from build123d import *

# Parameters (mm, degrees)
F4_START = 28
F4_DEPTH = 22
F6_START = -28
F5_W     = 60
F5_H     = 60
F6_DEPTH = 72


with BuildPart() as f2:
    # F1 (on Front) → F2 (revolve)
    with BuildSketch(Plane.XZ):
        with BuildLine():
            Line((-30, 0), (30, 0))
            ThreePointArc((30, 0), (0, 30), (-30, 0))
        make_face()
    revolve(axis=Axis((0, 0, 0), (1, 0, 0)))

    # F3 (on Top) → F4 (cut)
    with BuildSketch(Plane.XY.offset(F4_START)):
        Polygon((-9.1697992757, 6.1277179047), (-9.1697992757, -4.0975827724), (-6.1292964965, -5.6231399067), (-6.1292964965, 4.3796850368), (0, 7.6826182194), (5.4949265905, 4.3796850368), (5.4949265905, -2.3808549158), (-0.4257261462, -5.8186533861), (-4.6656387858, -3.3751989249), (-4.6656387858, -6.7009669729), (0, -9.1569181532), (8.5351010785, -4.193849396), (8.5351010785, 6.2439450994), (-0.4188895691, 11.2581793219), align=None)
        Polygon((-4.7212797217, 3.3881671261), (-4.7212797217, -1.4694901183), (0, -4.0975827724), (4.0084240027, -1.328688697), (4.0084240027, 3.3881671261), (0, 6.1423662119), align=None)
    extrude(amount=F4_DEPTH, mode=Mode.SUBTRACT)

    # F5 (on Top) → F6 (cut)
    with BuildSketch(Plane.XY.offset(F6_START)):
        with Locations((1.9770637155, -0.5929265171)):
            Rectangle(F5_W, F5_H)
    extrude(amount=-F6_DEPTH, mode=Mode.SUBTRACT)


solid = f2.part
Check sheet for the modelled part. Datum: model origin and axes. Units: mm. Round coordinates to 2 decimals unless told otherwise and drop trailing zeros. Loops run counter-clockwise (first coordinate to the right, second up) from the corner with the lowest first, then second, coordinate; pieces in that order, holes last.
1. Mould release check, pull along Y, two halves, no side actions. Record for faces 1 (the flat face through (-4.97, 8.59, 28.15)), 2 (the flat face through (0, 0, -28)), 3 (the flat face through (4.008, 1, 29)): released by +Y, released by -Y, zero draft, split by the parting line, or undercut.
2. Scan lines: probe 1 along Z at (x, y) = (-1, -3); probe 2 along Z at (x, y) = (19.5, -11); probe 3 along Y at (x, z) = (-16, 9.5). Record each from-to range of solid material in increasing order.
3. Sectioned sample at B-B on x = 3. Record the boundary of the cut face in (y, z), and give its area (3 significant figures).
4. Sectioned sample at C-C on z = -11. Record the boundary of the cut face in (x, y).
5. Gauge pin test, flat ends, axial feed: pin 1 Ø3 at (y, z) = (-7, -1) entering from +X; pin 2 Ø6 at (x, z) = (8.5, 1) entering from +Y; pin 3 Ø5 at (y, z) = (-7.5, 9.5) entering from +X. Record the tip position at first contact, or that the pin passes through.
6. Sectioned sample at D-D on y = -12. Record the boundary of the cut face in (x, z).
7. Sectioned sample at A-A on y = 2. Record the boundary of the cut face in (x, z), and give its area (3 significant figures).
Recorded:
1. face 1: undercut
1. face 2: zero draft
1. face 3: undercut
2. probe 1: z = -28 to 28
2. probe 2: z = -19.97 to 19.97
2. probe 3: y = -23.53 to 23.53
3. outline: (-10.34, -28) - (10.34, -28) arc R29.85 ccw to (9.34, 28.35) - (9.34, 28) - (5.88, 28) - (5.88, 29.26) arc R29.85 ccw to (4.08, 29.57) - (4.08, 28) - (-2.03, 28) - (-2.03, 29.78) arc R29.85 ccw to (-3.83, 29.6) - (-3.83, 28) - (-7.41, 28) - (-7.41, 28.91) arc R29.85 ccw to start
3. area: 2,760 mm2
4. outline: circle Ø55.82 at (0, 0)
5. pin 1: stops at x = 29.48
5. pin 2: stops at y = 29.48
5. pin 3: stops at x = 28.42
6. outline: circle Ø54.99 at (0, 0)
7. outline: (-10.58, -28) - (10.58, -28) arc R29.93 ccw to (8.54, 28.69) - (8.54, 28) - (5.49, 28) - (5.49, 29.42) arc R29.93 ccw to (4.01, 29.66) - (4.01, 28) - (-4.72, 28) - (-4.72, 29.56) arc R29.93 ccw to (-6.13, 29.3) - (-6.13, 28) - (-9.17, 28) - (-9.17, 28.49) arc R29.93 ccw to start
7. area: 2,770 mm2
